Verification items for the finished model (mm, model axes). Give positions to 0.01 mm unless a question says otherwise; leave off trailing zeros. Use CSV: the item, a comma, the result in double quotes.
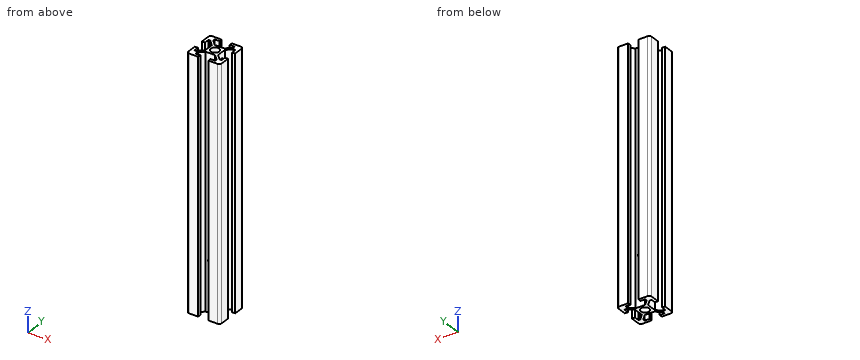
from build123d import *

# Parameters (mm, degrees)
SKETCH1_R           = 2.5
BOSS_EXTRUDE1_DEPTH = 150
FILLET1_R           = 1.47
SKETCH2_R           = 1.5
CUT_EXTRUDE1_DEPTH  = 151.974203094
SKETCH3_R           = 1.5
CUT_EXTRUDE2_DEPTH  = 151.974203194


with BuildPart() as part:
    # Sketch1 → Boss-Extrude1 (new body)
    with BuildSketch(Plane.XY):
        Polygon((2.860553032, 3.9), (6, 7.039446968), (6, 8.2), (3.1, 8.2), (3.1, 10), (10, 10), (10, 3.1), (8.2, 3.1), (8.2, 6), (7.039446968, 6), (3.9, 2.860553032), (3.9, 0), (3.9, -2.860553032), (7.039446968, -6), (8.2, -6), (8.2, -3.1), (10, -3.1), (10, -10), (3.1, -10), (3.1, -8.2), (6, -8.2), (6, -7.039446968), (2.860553032, -3.9), (0, -3.9), (-2.860553032, -3.9), (-6, -7.039446968), (-6, -8.2), (-3.1, -8.2), (-3.1, -10), (-10, -10), (-10, -3.1), (-8.2, -3.1), (-8.2, -6), (-7.039446968, -6), (-3.9, -2.860553032), (-3.9, 0), (-3.9, 2.860553032), (-7.039446968, 6), (-8.2, 6), (-8.2, 3.1), (-10, 3.1), (-10, 10), (-3.1, 10), (-3.1, 8.2), (-6, 8.2), (-6, 7.039446968), (-2.860553032, 3.9), (0, 3.9), align=None)
        Circle(SKETCH1_R, mode=Mode.SUBTRACT)
    extrude(amount=BOSS_EXTRUDE1_DEPTH)

    # Fillet1
    fillet1_edges = [part.edges().sort_by_distance(p)[0] for p in [
        (10, -10, 75),
        (-10, -10, 75),
        (-10, 10, 75),
        (10, 10, 75),
    ]]
    fillet(fillet1_edges, radius=FILLET1_R)

    # Sketch2 → Cut-Extrude1 (cut, through all)
    with BuildSketch(Plane.ZY.offset(3.9)):
        with Locations(Location((145, 0, 0), (0, 0, 270))):
            Circle(SKETCH2_R)
        with Locations(Location((135, 0, 0), (0, 0, 270))):
            Circle(SKETCH2_R)
        with Locations(Location((125, 0, 0), (0, 0, 270))):
            Circle(SKETCH2_R)
        with Locations(Location((30, 0, 0), (0, 0, 270))):
            Circle(SKETCH2_R)
    extrude(amount=-CUT_EXTRUDE1_DEPTH, mode=Mode.SUBTRACT)

    # Sketch3 → Cut-Extrude2 (cut, through all)
    with BuildSketch(Plane(origin=(0, 3.9, 0), x_dir=(1, 0, 0), z_dir=(0, 1, 0))):
        with Locations(Location((0, -30, 0), (0, 0, 180))):
            Circle(SKETCH3_R)
    extrude(amount=-CUT_EXTRUDE2_DEPTH, mode=Mode.SUBTRACT)


solid = part.part
(1) Depth check by flat-ended pin: pin 1 Ø3 at (y, z) = (1, 57) entering from +X; pin 2 Ø1.4 at (x, z) = (-9.5, 78) entering from +Y (3 decimals); pin 3 Ø2 at (x, z) = (0, 38.5) entering from -Y. Enter the tip coordinate at first touch or a pass-through.
Calculated:
pin 1,"stops at x = 3.9"
pin 2,"stops at y = 9.975"
pin 3,"stops at y = -3.9"
(2) Section check A-A on z = 30. Count the separate pieces of the cut face and the enclosed holes in it, plus the area to 3 significant figures.
Calculated:
separate pieces,"4"
enclosed holes,"0"
area,"148 mm²"
(3) Scan lines: L1, parallel to Y at x = 2.45, z = 145; L2, parallel to Y at x = -8.75, z = 102.5; L3, parallel to Y at x = -3.25, z = 122.5. Record each from-to range of solid material in increasing order. Write a range as from..to.
Calculated:
L1,"y = -3.9..-1.5, 1.5..3.9"
L2,"y = -9.98..-3.1, 3.1..9.98"
L3,"y = -10..-8.2, -4.29..4.29, 8.2..10"
